Verification items for the finished model (mm, model axes). A direction names the side the tool comes from. Coordinates: 2 decimals unless noted, no trailing zeros. Order: outer loops, then holes, each group sorted by start corner. A loop starts at its lowest first (then second) coordinate and runs counter-clockwise, first axis right, second up. Notation, with made-up numbers: M 55,-5.5 L 75,-5.5 A31 ccw 75,32.5 Z; hole C 67.5,81 d10. An arc over 180 degrees is marked long. Return JSON: item names as keys, results as strings. Group by question number.
Q1. Mould release check, pull along Y, two halves, no side actions. Record for faces 3 (the face through (0, 0, 49.5)), 4 (the face through (-15, 24, 19)), 5 (the face through (-29.97, 1.32, 35.21)): pulls with the +Y half, pulls with the -Y half, needs draft (parallel to the pull), parting line crosses it, or undercut.
Q2. Section check B-B, the plane y = 3. Enter the section's corners in (x, z), then the cut area to 3 significant figures.
Q3. Section check A-A, the plane x = 0. Enter the section's corners in (y, z), then the cut area to 3 significant figures.
Q4. Go/stop test with flat-tipped pins: pin 1 Ø2 at (y, z) = (-20, 34) entering from -X; pin 2 Ø2 at (y, z) = (-14.5, 23.5) entering from +X; pin 3 Ø10 at (x, y) = (9, 6.5) entering from -Z. Record where each tip stops, or that it passes through.
Q5. Section check C-C, the plane z = 32. Enter the section's corners in (x, y).
Q6. Access from +Z, -Z, +X, -X, +Y, -Y to the whole of each face (thin tool, end or side, straight path). Record for faces 1 (the face through (0, 0, 50)), 2 (the face through (13.38, -25.73, 19.51)).
Q7. Thickness scan on probe 1 along Y at (x, z) = (0, 35); probe 2 along X at (y, z) = (-19, 40); probe 3 along Z at (x, y) = (-13, -9.5). Record the ranges inside material, lowest first.
from build123d import *

# Parameters (mm, degrees)
SKETCH_R        = 30
PAD_DEPTH       = 20
SKETCH001_R     = 29
POCKET_DEPTH    = 1
SKETCH002_R     = 28
POCKET001_DEPTH = 19
SKETCH003_R     = 30
PAD001_DEPTH    = 31
SKETCH004_R     = 28
POCKET002_DEPTH = 29.5


with BuildPart() as body:
    # Sketch → Pad (new body)
    with BuildSketch(Plane.XY):
        Circle(SKETCH_R)
    extrude(amount=PAD_DEPTH)

    # Sketch001 → Pocket (cut)
    with BuildSketch(Plane.XY.offset(20)):
        Circle(SKETCH001_R)
    extrude(amount=-POCKET_DEPTH, mode=Mode.SUBTRACT)

    # Sketch002 (on Face3 of Pocket) → Pocket001 (cut)
    with BuildSketch(Plane.XY.offset(20)):
        Circle(SKETCH002_R)
    extrude(amount=-POCKET001_DEPTH, mode=Mode.SUBTRACT)


with BuildPart() as cut:
    # Sketch003 → Pad001 (new body)
    with BuildSketch(Plane.XY.offset(50)):
        Circle(SKETCH003_R)
    extrude(amount=-PAD001_DEPTH)

    # Sketch004 (on Face2 of Pad001) → Pocket002 (cut, symmetric)
    with BuildSketch(Plane.XY.offset(20)):
        Circle(SKETCH004_R)
    extrude(amount=POCKET002_DEPTH, both=True, mode=Mode.SUBTRACT)

    # Cut: cut Body
    add(body.part, mode=Mode.SUBTRACT)


solid = cut.part
Numbers:
{
 "1": {"face 3": "undercut", "face 4": "needs draft", "face 5": "parting line crosses it"},
 "2": {"outline": "M -29.85,20 L -28.84,20 L -28.84,19 L -27.84,19 L -27.84,49.5 L 27.84,49.5 L 27.84,19 L 28.84,19 L 28.84,20 L 29.85,20 L 29.85,50 L -29.85,50 Z", "area": "150 mm2"},
 "3": {"outline": "M -30,20 L -29,20 L -29,19 L -28,19 L -28,49.5 L 28,49.5 L 28,19 L 29,19 L 29,20 L 30,20 L 30,50 L -30,50 Z", "area": "150 mm2"},
 "4": {"pin 1": "stops at x = -23.22", "pin 2": "stops at x = 26.79", "pin 3": "stops at z = 49.5"},
 "5": {"outline": "C 0,0 d60; hole C 0,0 d56"},
 "6": {"face 1": "+Z, +X, -X, +Y, -Y", "face 2": "-Z"},
 "7": {"probe 1": "y = -30 to -28, 28 to 30", "probe 2": "x = -23.22 to -20.57, 20.57 to 23.22", "probe 3": "z = 49.5 to 50"}
}
